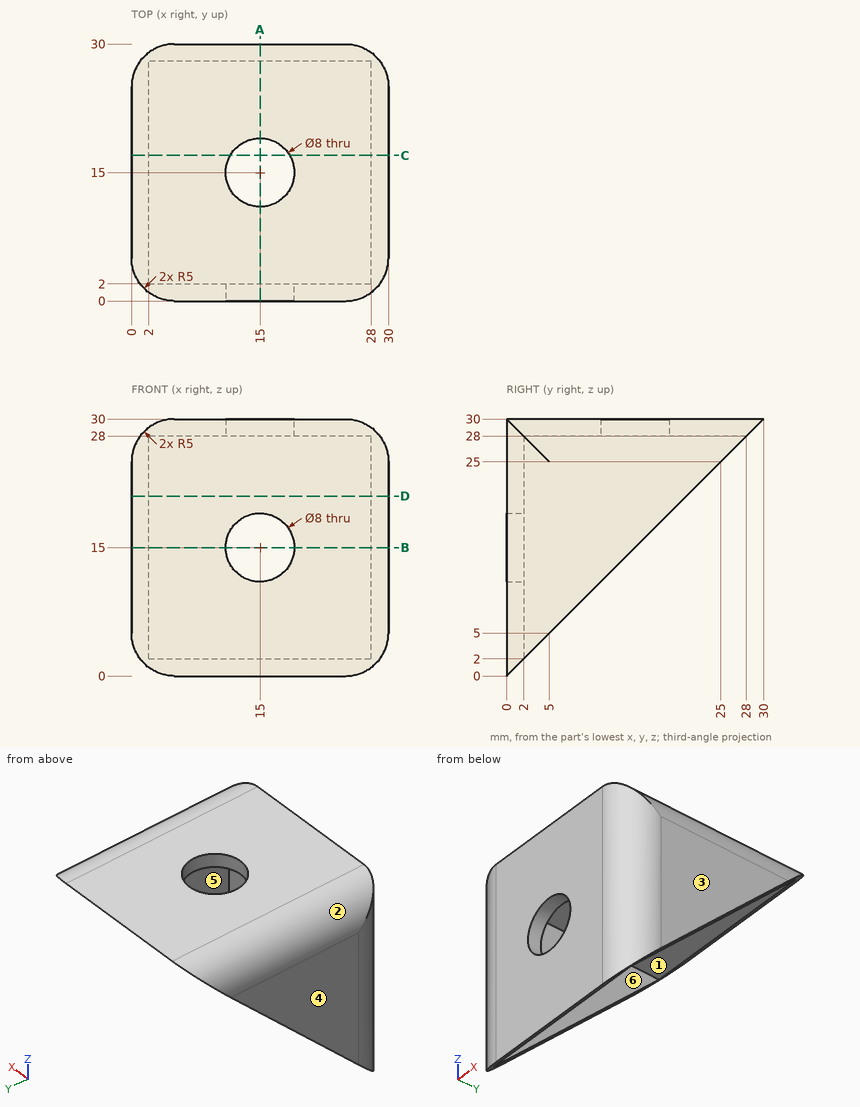
Answer from the drawing. Dimensions are ordinates in mm from the lowest x, y and z of the part. A direction names the side the tool comes from. Coordinates: 2 decimals unless noted, no trailing zeros. Loops run counter-clockwise (first coordinate to the right, second up) from the corner with the lowest first, then second, coordinate; pieces in that order, holes last. Notation, with made-up numbers: (84, 23.5) -> (108, 23.5) arc R20 cw to (108, 43.5) -> close; hole circle Ø9 at (5.25, 55.25). An arc over 180 degrees is marked (long way). Return JSON: item names as keys, results as strings.
Item 1: Find section B-B (z = 15). Determine the outline of the cut face in (x, y), plus the area to 3 significant figures.
Answers:
{"outline": "(0, 5) arc R5 ccw to (5, 0) -> (11, 0) -> (11, 2) -> (2, 2) -> (2, 15) -> (0, 15) -> close; (19, 0) -> (25, 0) arc R5 ccw to (30, 5) -> (30, 15) -> (28, 15) -> (28, 2) -> (19, 2) -> close", "area": "85.3 mm2"}
Item 2: Flat-ended cylindrical pins translate along their axes: P1, Ø3, axis at x = 16.5, y = 24, coming from the -Z side; P2, Ø10.5, axis at x = 15, z = 15, coming from the +Y side. Find the tip coordinate at first contact, or state that the pin passes through.
Answers:
{"P1": "stops at z = 28", "P2": "stops at y = 2"}
Item 3: Find section A-A (x = 15). Determine the outline of the cut face in (y, z), plus the area to 3 significant figures.
Answers:
{"outline": "(0, 0) -> (2, 2) -> (2, 11) -> (0, 11) -> close; (0, 19) -> (2, 19) -> (2, 28) -> (11, 28) -> (11, 30) -> (0, 30) -> close; (19, 28) -> (28, 28) -> (30, 30) -> (19, 30) -> close", "area": "80.0 mm2"}
Item 4: For a pull along X with two mould halves and no side action, classify the marked faces 3, 4, 5 and 6 as +X half, -X half, draft (parallel to the pull), parting line (faces both ways), or undercut.
Answers:
{"face 3": "+X half", "face 4": "-X half", "face 5": "undercut", "face 6": "undercut"}
Item 5: Find section C-C (y = 17). Determine the outline of the cut face in (x, z), plus the area to 3 significant figures.
Answers:
{"outline": "(0, 17) -> (2, 17) -> (2, 28) -> (11.54, 28) -> (11.54, 30) -> (5, 30) arc R5 ccw to (0, 25) -> close; (18.46, 28) -> (28, 28) -> (28, 17) -> (30, 17) -> (30, 25) arc R5 ccw to (25, 30) -> (18.46, 30) -> close", "area": "79.4 mm2"}
Item 6: Find the intervals of material crossed by probe 1 along Z at (x, y) = (6.5, 19); probe 2 along X at (y, z) = (5.5, 10); probe 3 along Z at (x, y) = (15, 1.5), in increasing order.
Answers:
{"probe 1": "z = 28 to 30", "probe 2": "x = 0 to 2, 28 to 30", "probe 3": "z = 1.5 to 11, 19 to 30"}
Item 7: For the marked faces 1 and 2, determine the directions among +Z, -Z, +X, -X, +Y, -Y from which every point of the face is accessible in a straight line to the end or side of a thin tool.
Answers:
{"face 1": "-Z, +Y", "face 2": "+Z, -X, +Y, -Y"}
Item 8: Find section D-D (z = 21). Determine the outline of the cut face in (x, y).
Answers:
{"outline": "(0, 5) arc R5 ccw to (5, 0) -> (25, 0) arc R5 ccw to (30, 5) -> (30, 21) -> (28, 21) -> (28, 2) -> (2, 2) -> (2, 21) -> (0, 21) -> close"}
